from build123d import *

# Parameters (mm, degrees)
BOSS_EXTRUDE1_DEPTH = 20
SHELL1_T            = -3
SKETCH3_R           = 9.972851257
SKETCH3_R_2         = 7.972851257
BOSS_EXTRUDE2_DEPTH = 18
SKETCH4_W           = 45
SKETCH4_H           = 16
CUT_EXTRUDE2_DEPTH  = 98


with BuildPart() as part:
    # Sketch1 → Boss-Extrude1 (new body)
    with BuildSketch(Plane(origin=(0, 0, 0), x_dir=(1, 0, 0), z_dir=(0, 1, 0))):
        with BuildLine():
            Line((-80, -50), (80, -50))
            ThreePointArc((80, -50), (87.071067812, -47.071067812), (90, -40))
            Line((90, -40), (90, 40))
            ThreePointArc((90, 40), (87.071067812, 47.071067812), (80, 50))
            Line((80, 50), (-80, 50))
            ThreePointArc((-80, 50), (-87.071067812, 47.071067812), (-90, 40))
            Line((-90, 40), (-90, -40))
            ThreePointArc((-90, -40), (-87.071067812, -47.071067812), (-80, -50))
        make_face()
    extrude(amount=BOSS_EXTRUDE1_DEPTH)

    # Shell1
    shell1_openings = [part.faces().sort_by_distance(p)[0] for p in [
        (0, 20, 0),
    ]]
    offset(amount=SHELL1_T, openings=shell1_openings, kind=Kind.INTERSECTION)

    # Sketch3 → Boss-Extrude2 (add)
    # profile 1 of 4: a face of its own
    with BuildSketch(Plane(origin=(0, 3, 0), x_dir=(1, 0, 0), z_dir=(0, 1, 0))):
        with Locations(Location((-70, 30, 0), (0, 0, 90))):
            Circle(SKETCH3_R)
        with Locations(Location((-70, 30, 0), (0, 0, 270))):
            Circle(SKETCH3_R_2, mode=Mode.SUBTRACT)
    # profile 2 of 4: a face of its own
    with BuildSketch(Plane(origin=(0, 3, 0), x_dir=(1, 0, 0), z_dir=(0, 1, 0))):
        with Locations(Location((70, 30, 0), (0, 0, 90))):
            Circle(SKETCH3_R)
        with Locations(Location((70, 30, 0), (0, 0, 90))):
            Circle(SKETCH3_R_2, mode=Mode.SUBTRACT)
    # profile 3 of 4: a face of its own
    with BuildSketch(Plane(origin=(0, 3, 0), x_dir=(1, 0, 0), z_dir=(0, 1, 0))):
        with Locations(Location((70, -30, 0), (0, 0, 90))):
            Circle(SKETCH3_R)
        with Locations(Location((70, -30, 0), (0, 0, 270))):
            Circle(SKETCH3_R_2, mode=Mode.SUBTRACT)
    # profile 4 of 4: a face of its own
    with BuildSketch(Plane(origin=(0, 3, 0), x_dir=(1, 0, 0), z_dir=(0, 1, 0))):
        with Locations(Location((-70, -30, 0), (0, 0, 90))):
            Circle(SKETCH3_R)
        with Locations(Location((-70, -30, 0), (0, 0, 90))):
            Circle(SKETCH3_R_2, mode=Mode.SUBTRACT)
    extrude(amount=BOSS_EXTRUDE2_DEPTH)

    # Sketch4 → Cut-Extrude2 (cut)
    with BuildSketch(Plane.XY.offset(50)):
        with Locations((-32.5, 10)):
            Rectangle(SKETCH4_W, SKETCH4_H)
    extrude(amount=-CUT_EXTRUDE2_DEPTH, mode=Mode.SUBTRACT)


solid = part.part
Model file for the job. Use its own axes, mm. A direction names the side the tool comes from. Give positions to 0.01 mm unless a question says otherwise; leave off trailing zeros. Loops run counter-clockwise (first coordinate to the right, second up) from the corner with the lowest first, then second, coordinate; pieces in that order, holes last.
Item 1: Slice it at D-D (z = 5). Write the cut outline in (x, y).
Check values:
outline: (-90, 0) - (90, 0) - (90, 20) - (87, 20) - (87, 3) - (-10, 3) - (-10, 2) - (-55, 2) - (-55, 3) - (-87, 3) - (-87, 20) - (-90, 20) - close
Item 2: Mould opens along Z. For faces 4 (the face through (-1, 0, -1)), 5 (the face through (-63.932, 11.874, -22.086)), 6 (the face through (62.095, 11.874, -28.962)), 7 (the face through (-87.15, 9.86, 46.99)) say: +Z half, -Z half, draft (parallel to the pull), parting line (faces both ways), or undercut.
Check values:
face 4: draft
face 5: undercut
face 6: undercut
face 7: +Z half
Item 3: Drill centre lines: line 1 along X through (y, z) = (17.75, 30); line 2 along X through (y, z) = (12.25, 14); line 3 along X through (y, z) = (9, 32). Where is each one in solid material? Low to high.
Check values:
line 1: x = -90 to -87, -79.97 to -77.97, -62.03 to -60.03, 60.03 to 62.03, 77.97 to 79.97, 87 to 90
line 2: x = -90 to -87, 87 to 90
line 3: x = -90 to -87, -79.77 to -77.72, -62.28 to -60.23, 60.23 to 62.28, 77.72 to 79.77, 87 to 90
Item 4: Slice it at C-C (x = 70). Write the cut outline in (y, z).
Check values:
outline: (0, -50) - (20, -50) - (20, -47) - (3, -47) - (3, -39.97) - (21, -39.97) - (21, -37.97) - (3, -37.97) - (3, -22.03) - (21, -22.03) - (21, -20.03) - (3, -20.03) - (3, 20.03) - (21, 20.03) - (21, 22.03) - (3, 22.03) - (3, 37.97) - (21, 37.97) - (21, 39.97) - (3, 39.97) - (3, 47) - (20, 47) - (20, 50) - (0, 50) - close
Item 5: Slice it at A-A (y = 9.5). Give the number of separate pieces and of enclosed holes in the cut face, plus the area to 3 significant figures.
Check values:
separate pieces: 5
enclosed holes: 4
area: 1,870 mm2
Item 6: Which spindle directions (+Z, -Z, +X, -X, +Y, -Y) get a long thin tool onto all of the face, cutting with end or side? Do faces 1 (the face through (-55, 2.3, 15.7)), 2 (the face through (-87, 11, -1)), 3 (the face through (-61.9, 21, 30.8)). Say none if no direction does.
Check values:
face 1: +Z
face 2: +Y
face 3: +Z, -Z, +X, -X, +Y
Item 7: Drop flat-ended pins along their axis: P1, Ø13, axis at x = -70, z = -30, coming from the +Y side; P2, Ø5, axis at x = -20, z = -34.5, coming from the +Y side. Give the stop position or say it passes through.
Check values:
P1: stops at y = 3
P2: stops at y = 2
Item 8: Slice it at B-B (z = 30). Write the cut outline in (x, y), plus the area to 3 significant figures.
Check values:
outline: (-90, 0) - (90, 0) - (90, 20) - (87, 20) - (87, 3) - (79.97, 3) - (79.97, 21) - (77.97, 21) - (77.97, 3) - (62.03, 3) - (62.03, 21) - (60.03, 21) - (60.03, 3) - (-10, 3) - (-10, 2) - (-55, 2) - (-55, 3) - (-60.03, 3) - (-60.03, 21) - (-62.03, 21) - (-62.03, 3) - (-77.97, 3) - (-77.97, 21) - (-79.97, 21) - (-79.97, 3) - (-87, 3) - (-87, 20) - (-90, 20) - close
area: 741 mm2
